Can you work these out from the model? Positions are in its coordinate system, mm. A direction names the side the tool comes from. Round coordinates to 2 decimals unless told otherwise and drop trailing zeros. Write each loop counter-clockwise with the first axis right and the second up, starting at its lowest first coordinate (ties: lowest second). Pieces come first, ordered by that corner, then holes.
Q1. If we section it at B-B (y = 2.25): Please give me the cut outline in (x, z).
Q2. If we section it at C-C (x = 10): Please give me the cut outline in (y, z).
Q3. If we section it at A-A (z = 0.9): Please give me the cut outline in (x, y), plus the area to 3 significant figures.
Q4. For faces 1 (the flat face through (50, 17, 1)), 2 (the flat face through (-1, 17, 1)), 3 (the flat face through (24, 22, 1)), which set-ups out of +Z, -Z, +X, -X, +Y, -Y let a thin tool reach every point of the face, with its end or its side?
Q5. Please list where these lines run through material, in increasing order: line 1 along X through (y, z) = (22.5, 0.75); line 2 along X through (y, z) = (10.25, 2.6); line 3 along Y through (x, z) = (26, 0.7).
Q6. I'm going to push flat-ended pins straight in: pin 1 Ø1.5 at (y, z) = (14.5, 1) entering from -X; pin 2 Ø1.5 at (x, z) = (40.5, 2) entering from -Y. Where does each tip first touch, or does it pass through?
Q7. We'd pull the mould along X, two halves only. Please class faces 4 (the flat face through (0, 14, 1)), 5 (the flat face through (49, 10, 1)), 6 (the flat face through (2, 23, 1)): +X half, -X half, draft (parallel to the pull), parting line (faces both ways), or undercut.
Autodesk Inventor part; units mm, degrees
ref_plane "YZ Plane" through (0, 0, 0) normal (1, 0, 0) x (0, 1, 0)
ref_plane "XZ Plane" through (0, 0, 0) normal (0, 1, 0) x (-1, 0, 0)
ref_plane "XY Plane" through (0, 0, 0) normal (0, 0, 1) x (1, 0, 0)
sketch "Sketch1" plane through (0, 0, 0) normal (0, 0, 1) x (1, 0, 0)
  line L0 (39, 0) -> (25, 0)
  line L1 (25, 0) -> (24, 0)
  line L2 (24, 11) -> (24, 0)
  line L3 (16.5, 11) -> (24, 11)
  line L4 (-3, 11) -> (16.5, 11)
  line L5 (0, 17) -> (0, 25)
  line L6 (49, 25) -> (49, 17)
  line L7 (49, 17) -> (52, 17)
  line L8 (52, 25) -> (52, 17)
  line L9 (49, 25) -> (52, 25)
  line L10 (49, 17) -> (49, 0)
  line L11 (39, 3) -> (49, 3)
  line L12 (39, 0) -> (39, 3)
  line L13 (0, 17) -> (0, 11)
  line L14 (2, 22) -> (2, 25)
  line L15 (2, 25) -> (0, 25)
  line L16 (0, 25) -> (0, 20)
  line L17 (47, 22) -> (47, 25)
  line L18 (47, 25) -> (49, 25)
  line L19 (0, 17) -> (0, 25)
  line L20 (0, 25) -> (-3, 25)
  line L21 (-3, 17) -> (-3, 25)
  line L22 (0, 17) -> (-3, 17)
  line L23 (2, 22) -> (47, 22)
  point P0 (0, 0)
  dimension "d2" = 5
  dimension "d4" = 5
  dimension "d5" = 3
extrude "Extrusion1" add sketch "Sketch1" along normal blind 3
properties part number "SideBottomNM" material "Acrylic, Clear"
A:
1. outline: (24, 0) - (39, 0) - (39, 3) - (24, 3) - close
2. outline: (11, 0) - (22, 0) - (22, 3) - (11, 3) - close
3. outline: (-3, 17) - (0, 17) - (0, 11) - (24, 11) - (24, 0) - (39, 0) - (39, 3) - (49, 3) - (49, 17) - (52, 17) - (52, 25) - (47, 25) - (47, 22) - (2, 22) - (2, 25) - (-3, 25) - close
3. area: 844 mm2
4. face 1: +Z, -Z, +X, -Y
4. face 2: +Z, -Z, -X, -Y
4. face 3: +Z, -Z, +Y
5. line 1: x = -3 to 2, 47 to 52
5. line 2: x = 24 to 49
5. line 3: y = 0 to 22
6. pin 1: stops at x = 0
6. pin 2: stops at y = 3
7. face 4: -X half
7. face 5: +X half
7. face 6: undercut
